For this review, take the finished solid that the model builds, in its own axes (mm). A direction names the side the tool comes from. Round coordinates to 2 decimals unless told otherwise and drop trailing zeros. Loops run counter-clockwise (first coordinate to the right, second up) from the corner with the lowest first, then second, coordinate; pieces in that order, holes last.
1. Clearance check with flat-ended pins moving along their axes: pin 1 Ø1.5 at (y, z) = (-8, 11.5) entering from +X; pin 2 Ø8 at (y, z) = (-30, 9) entering from +X; pin 3 Ø2 at (x, z) = (11.5, 1) entering from -Y; pin 4 Ø1.8 at (x, z) = (11.5, 8) entering from -Y. State where each tip first meets the part, or that it passes through.
2. To check wall thickness, follow line 1 along Y through (x, z) = (13.5, 1.25); line 2 along Z through (x, y) = (3, -31); line 3 along Y through (x, z) = (3.25, 9). State the ranges of each line that lie inside material, in increasing order.
3. Consider section A-A on y = -4. State the section outline as (x, z) points, then the cut area to 3 significant figures.
4. Consider section B-B on x = 3.75. State the section outline as (y, z) points.
5. Consider section D-D on z = 9. State the section outline as (x, y) points, then the cut area to 3 significant figures.
6. Draft analysis for pull direction Y (two halves, no side actions). For faces 1 (the cylindrical face through (4.93, -14.8, 13.41)), 2 (the cylindrical face through (5.07, -15.554, 3.962)), 3 (the flat face through (11.48, -7.49, 7.71)), state which applies: released by +Y, released by -Y, zero draft, split by the parting line, or undercut.
7. Consider section C-C on y = -27. State the section outline as (x, z) points, then the cut area to 3 significant figures.
8. Tool access review of faces 4 (the flat face through (11, -19.599, 9)), 5 (the flat face through (5, -14.599, 9)), 6 (the flat face through (3, -26, 4.124)): name each direction out of +Z, -Z, +X, -X, +Y, -Y from which nothing blocks a thin tool from reaching the whole face with its end or side.
from build123d import *

# Parameters (mm, degrees)
EXTRUDE_THIN1_DEPTH = 15
SKETCH4_OUTSIDE_W   = 26.324
SKETCH4_OUTSIDE_H   = 51.391
CUT_EXTRUDE1_DEPTH  = 45.568245566
CUT_EXTRUDE2_DEPTH  = 3
SKETCH7_R           = 1.75
SKETCH7_R_2         = 0.75
CUT_EXTRUDE3_DEPTH  = 43.275324346
FILLET1_R           = 4
FILLET2_R           = 2
FILLET3_R           = 2


with BuildPart() as part:
    # Sketch3 → Extrude-Thin1 (new body)
    with BuildSketch(Plane(origin=(0, 0, 0), x_dir=(0, 0, -1), z_dir=(1, 0, 0))):
        Polygon((-4.385708038, 2.401159095), (-14.124404563, -15.386533403), (-14.124404563, -37.665690546), (-4.124404563, -37.665690546), (-4.124404563, -17.944847689), (4.385708038, -2.401159095), align=None)
    extrude(amount=EXTRUDE_THIN1_DEPTH)

    # Sketch4 outside → Cut-Extrude1 (cut, through all)
    with BuildSketch(Plane.XY.offset(14.124404563)):
        with Locations((7.5, -17.6325)):
            Rectangle(SKETCH4_OUTSIDE_W, SKETCH4_OUTSIDE_H)
        Polygon((15, 2.401159095), (10, 2.401159095), (10, -14.598840905), (0, -14.598840905), (0, -37.665690546), (7, -37.665690546), (7, -19.598840905), (15, -19.598840905), align=None, mode=Mode.SUBTRACT)
    extrude(amount=-CUT_EXTRUDE1_DEPTH, mode=Mode.SUBTRACT)

    # Sketch6 → Cut-Extrude2 (cut)
    with BuildSketch(Plane.ZY.offset(-10)):
        with BuildLine():
            Line((-0.921976714, -6.081964697), (5.150298165, -14.851265553))
            Line((5.150298165, -14.851265553), (9.736888227, -12.340124285))
            Line((9.736888227, -12.340124285), (5.620547292, -2.499956755))
            ThreePointArc((5.620547292, -2.499956755), (0.360173864, -0.657856206), (-0.921976714, -6.081964697))
        make_face()
    extrude(amount=-CUT_EXTRUDE2_DEPTH, mode=Mode.SUBTRACT)

    # Sketch7 → Cut-Extrude3 (cut, through all)
    with BuildSketch(Plane.ZY.offset(-13)):
        with Locations(Location((2.161043186, -3.947137235, 0), (0, 0, 270))):
            Circle(SKETCH7_R)
        with Locations(Location((4.562202281, -8.332845273, 0), (0, 0, 270))):
            Circle(SKETCH7_R_2)
        with Locations(Location((6.483129558, -11.841411704, 0), (0, 0, 270))):
            Circle(SKETCH7_R_2)
    extrude(amount=-CUT_EXTRUDE3_DEPTH, mode=Mode.SUBTRACT)

    # Fillet1
    fillet1_edges = [part.edges().sort_by_distance(p)[0] for p in [
        (3.5, -37.665690546, 4.124404563),
        (3.5, -37.665690546, 14.124404563),
        (12.5, 2.401159095, 4.385708038),
        (12.5, -2.401159095, -4.385708038),
    ]]
    fillet(fillet1_edges, radius=FILLET1_R)

    # Fillet2
    # the kernel refuses this fillet: 2 mm, written as the material it takes off along each edge
    with BuildSketch(Plane(origin=(7, -19.598840905, 14.124404563), x_dir=(0, 1, 0), z_dir=(1, 0, 0))) as fillet2_piece_1:
        with BuildLine():
            CenterArc((FILLET2_R, -FILLET2_R), FILLET2_R, 90, 90)
            Line((0, -FILLET2_R), (-FILLET2_R * 0.02, -FILLET2_R))
            Line((-FILLET2_R * 0.02, -FILLET2_R), (-FILLET2_R * 0.02, FILLET2_R * 0.02))
            Line((-FILLET2_R * 0.02, FILLET2_R * 0.02), (FILLET2_R, FILLET2_R * 0.02))
            Line((FILLET2_R, FILLET2_R * 0.02), (FILLET2_R, 0))
        make_face()
    extrude(amount=13, mode=Mode.SUBTRACT)
    with BuildSketch(Plane(origin=(7, -19.598840905, 4.124404563), x_dir=(0, 1, 0), z_dir=(1, 0, 0))) as fillet2_piece_2:
        with BuildLine():
            CenterArc((2, 1.969842457), FILLET2_R, 180, 80.037511241)
            Line((0, 1.969842457), (-0.04, 1.969842457))
            Line((-0.04, 1.969842457), (-0.04, 0))
            Line((-0.04, 0), (0, -0.04))
            ThreePointArc((0, -0.04), (0.826996608, -0.04), (1.64707308, -0.039396849))
            Line((1.64707308, -0.039396849), (1.653993216, 0))
        make_face()
    extrude(amount=12.924606142, mode=Mode.SUBTRACT)

    # Fillet3
    # the kernel refuses this fillet: 2 mm, written as the material it takes off along each edge
    with BuildSketch(Plane(origin=(10, -14.598840905, 2.292478098), x_dir=(0, -0.8771416076820373, 0.48023181909674706), z_dir=(-1, 0, 0))) as fillet3_piece_1:
        with BuildLine():
            CenterArc((FILLET3_R * 1.68756310969, FILLET3_R), FILLET3_R, 151.299456423, 118.700543577)
            Line((FILLET3_R * 0.810421502006, FILLET3_R * 1.4802318191), (FILLET3_R * 0.792878669852, FILLET3_R * 1.48983645548))
            Line((FILLET3_R * 0.792878669852, FILLET3_R * 1.48983645548), (-FILLET3_R * 0.0337512621938, -FILLET3_R * 0.02))
            Line((-FILLET3_R * 0.0337512621938, -FILLET3_R * 0.02), (FILLET3_R * 1.68756310969, -FILLET3_R * 0.02))
            Line((FILLET3_R * 1.68756310969, -FILLET3_R * 0.02), (FILLET3_R * 1.68756310969, 0))
        make_face()
    extrude(amount=18.437815548, mode=Mode.SUBTRACT)
    with BuildSketch(Plane(origin=(-2.898590554, -14.598840905, 13.693145803), x_dir=(0, -0.8771416076820384, 0.48023181909674506), z_dir=(1, 0, 0))) as fillet3_piece_2:
        with BuildLine():
            CenterArc((1.19748505, 1.97745339), FILLET3_R, 208.700543577, 52.688089319)
            Line((-0.556798166, 1.016989751), (-0.59188383, 0.997780479))
            Line((-0.59188383, 0.997780479), (-0.035085664, -0.019209273))
            Line((-0.035085664, -0.019209273), (0, -0.04))
            ThreePointArc((0, -0.04), (0.449011022, -0.04), (0.892032783, -0.039549068))
            Line((0.892032783, -0.039549068), (0.898022043, 0))
        make_face()
    extrude(amount=12.898590554, mode=Mode.SUBTRACT)


solid = part.part
Resolved:
1. pin 1: passes through
1. pin 2: stops at x = 7
1. pin 3: stops at y = -14.06
1. pin 4: stops at y = -19.6
2. line 1: y = -12.69 to -5.44, -2.45 to 0.66
2. line 2: z = 4.12 to 14.12
2. line 3: y = -37.67 to -14.6
3. outline: (10, -2.96) - (15, -2.96) - (15, 0.41) - (13, 0.41) - (13, -1.59) - (10, -1.59) - close; (10, 6.25) - (13, 6.25) - (13, 3.91) - (15, 3.91) - (15, 7.89) - (10, 7.89) - close
3. area: 23.7 mm2
4. outline: (-37.67, 8.12) arc R4 ccw to (-33.67, 4.12) - (-17.94, 4.12) - (-17.56, 3.91) arc R2 ccw to (-14.6, 5.67) - (-14.6, 12.53) arc R2 ccw to (-15.39, 14.12) - (-33.67, 14.12) arc R4 ccw to (-37.67, 10.12) - close
5. outline: (0, -37.67) - (7, -37.67) - (7, -19.6) - (15, -19.6) - (15, -6.03) - (10, -6.03) - (10, -10.58) - (13, -10.58) - (13, -12.74) - (10, -12.74) - (10, -14.6) - (0, -14.6) - close
5. area: 238 mm2
6. face 1: released by +Y
6. face 2: split by the parting line
6. face 3: undercut
7. outline: (0, 4.12) - (7, 4.12) - (7, 14.12) - (0, 14.12) - close
7. area: 70.0 mm2
8. face 4: +Z, -Z, +X, -Y
8. face 5: +Z, -Z, -X, +Y
8. face 6: -Z, +X, -X, -Y
